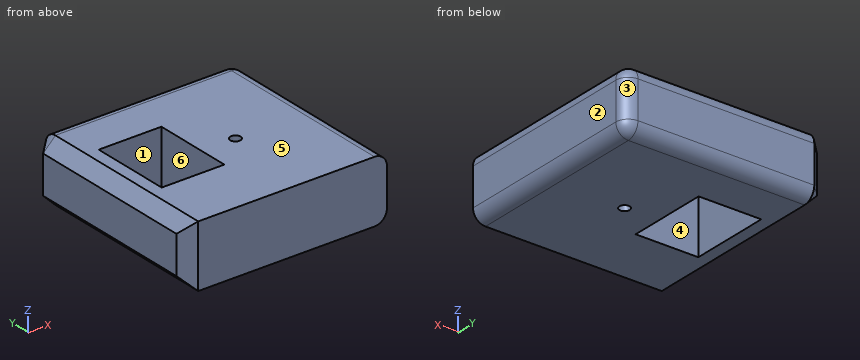
```python
from build123d import *

# Parameters (mm, degrees)
F0_W     = 82.0379033685
F0_H     = 79.8256471753
F1_DEPTH = 25.4
F3_D     = 4.2
F4_R     = 5.08
F5_R     = 5.08
F6_R     = 5.08
F7_W     = 25.5733272061
F7_H     = 32.9347681254
F8_DEPTH = 25.4
F9_SIZE  = 5


with BuildPart() as f1:
    # F0 (on Top) → F1 (new body)
    with BuildSketch(Plane.XY):
        with Locations((41.0189516842, 39.9128235877)):
            Rectangle(F0_W, F0_H)
    extrude(amount=F1_DEPTH)

    # F3 (through all)
    with Locations(Plane.XY.offset(25.4)):
        with Locations((49.3793413043, 37.4442487955)):
            Hole(F3_D / 2)

    # F4
    f4_edges = [f1.edges().sort_by_distance(p)[0] for p in [
        (82.037903, 79.825647, 12.7),
    ]]
    fillet(f4_edges, radius=F4_R)

    # F5
    f5_edges = [f1.edges().sort_by_distance(p)[0] for p in [
        (82.037903, 37.372824, 0),
    ]]
    fillet(f5_edges, radius=F5_R)

    # F6
    f6_edges = [f1.edges().sort_by_distance(p)[0] for p in [
        (38.478952, 79.825647, 25.4),
    ]]
    fillet(f6_edges, radius=F6_R)

    # F7 (on face) → F8 (cut)
    with BuildSketch(Plane.XY.offset(25.4)):
        with Locations((22.7667321451, 41.983817704)):
            Rectangle(F7_W, F7_H)
    extrude(amount=-F8_DEPTH, mode=Mode.SUBTRACT)

    # F9
    f9_edges = [f1.edges().sort_by_distance(p)[0] for p in [
        (0, 79.825647, 12.7),
        (0, 78.33775, 23.912102),
        (0, 78.33775, 1.487898),
        (0, 37.372824, 25.4),
        (0, 37.372824, 0),
        (0, 0, 12.7),
    ]]
    chamfer(f9_edges, length=F9_SIZE)


solid = f1.part
```
Check sheet for the modelled part. Datum: model origin and axes. Units: mm. Face numbers are marked on the shaded views. A direction names the side the tool comes from. Round coordinates to 2 decimals unless told otherwise and drop trailing zeros. Loops run counter-clockwise (first coordinate to the right, second up) from the corner with the lowest first, then second, coordinate; pieces in that order, holes last. Notation, with made-up numbers: M 27,-26.75 L 73,-26.75 A36 ccw 73,12.25 Z; hole C 79,28.5 d10. An arc over 180 degrees is marked long. Answer as a JSON object with one key per item and string values.
1. Section check C-C (y = 11). Record the boundary of the cut face in (x, z), plus the area to 3 significant figures.
Reply:
{"outline": "M 0,5 L 5,0 L 76.96,0 A5.08 ccw 82.04,5.08 L 82.04,20.32 A5.08 ccw 76.96,25.4 L 5,25.4 L 0,20.4 Z", "area": "2,050 mm²"}
2. Mould release check, pull along Y, two halves, no side actions. Record for the marked faces 3, 4, 5 and 6: pulls with the +Y half, pulls with the -Y half, needs draft (parallel to the pull), parting line crosses it, or undercut.
Reply:
{"face 3": "pulls with the +Y half", "face 4": "undercut", "face 5": "needs draft", "face 6": "undercut"}
3. Scan lines: line 1 (X direction, y = 29, z = 15); line 2 (Y direction, x = 27.5, z = 12); line 3 (Y direction, x = 33, z = 2). Record each from-to range of solid material in increasing order.
Reply:
{"line 1": "x = 0 to 9.98, 35.55 to 82.04", "line 2": "y = 0 to 25.52, 58.45 to 79.83", "line 3": "y = 0 to 25.52, 58.45 to 78.79"}
4. Section check D-D (z = 9.75). Record the boundary of the cut face in (x, y), plus the area to 3 significant figures.
Reply:
{"outline": "M 0,5 L 5,0 L 82.04,0 L 82.04,74.75 A5.08 ccw 76.96,79.83 L 5,79.83 L 0,74.83 Z; hole M 9.98,25.52 L 35.55,25.52 L 35.55,58.45 L 9.98,58.45 Z; hole C 49.38,37.44 d4.2", "area": "5,660 mm²"}
5. Access from +Z, -Z, +X, -X, +Y, -Y to the whole of each face (thin tool, end or side, straight path). Record for the marked faces 1 and 2.
Reply:
{"face 1": "+Z, -Z", "face 2": "+Z, -Z, +X, +Y, -Y"}
6. Section check B-B (y = 30). Record the boundary of the cut face in (x, z).
Reply:
{"outline": "M 0,5 L 5,0 L 9.98,0 L 9.98,25.4 L 5,25.4 L 0,20.4 Z; M 35.55,0 L 76.96,0 A5.08 ccw 82.04,5.08 L 82.04,20.32 A5.08 ccw 76.96,25.4 L 35.55,25.4 Z"}
7. Section check A-A (x = 22). Record the boundary of the cut face in (y, z), plus the area to 3 significant figures.
Reply:
{"outline": "M 0,0 L 25.52,0 L 25.52,25.4 L 0,25.4 Z; M 58.45,0 L 74.75,0 A5.08 ccw 79.83,5.08 L 79.83,20.32 A5.08 ccw 74.75,25.4 L 58.45,25.4 Z", "area": "1,180 mm²"}
